The listing builds one solid part. Answer for the finished solid, in the listing's coordinates (mm). Face numbers are marked on the shaded views. A direction names the side the tool comes from. Give positions to 0.01 mm unless a question says otherwise; leave off trailing zeros. Order: outer loops, then holes, each group sorted by start corner. A loop starts at its lowest first (then second) coordinate and runs counter-clockwise, first axis right, second up. Notation, with made-up numbers: (64.25, 54) - (103.25, 54) arc R24 ccw to (103.25, 83) - close; hole circle Ø1 at (-9, 78.25). An arc over 180 degrees is marked (long way). Use CSV: the item, a comma, the result in double quotes.
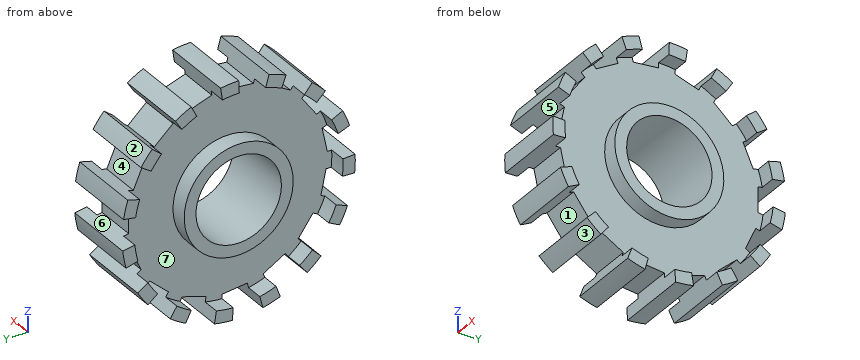
```python
from build123d import *

# Parameters (mm, degrees)
CUT_EXTRUDE3_DEPTH = 16
CIRPATTERN1_COUNT  = 15


with BuildPart() as part:
    # Sketch1 → Revolve1 (revolve)
    with BuildSketch(Plane.XY, mode=Mode.PRIVATE) as revolve1_sk:
        Polygon((0, 5.778414329), (-10, 5.778414329), (-10, 7.373034886), (-7.662379617, 7.373034886), (-7.662379617, 14.122184027), (-10, 14.122184027), (-10, 15.778414329), (0, 15.778414329), (0, 14.122184027), (-2.126486554, 14.122184027), (-2.126486554, 7.373034886), (0, 7.373034886), align=None)
    revolve(revolve1_sk.sketch.rotate(Axis((0, 0, 0), (-1, 0, 0)), 90), axis=Axis((0, 0, 0), (-1, 0, 0)))

    # Sketch2 → Cut-Extrude3 (cut)
    with BuildSketch(Plane(origin=(0, 0, 0), x_dir=(0, 0, -1), z_dir=(1, 0, 0))):
        Polygon((-2.776343501, 17.284448499), (-2.119655167, 13.369575739), (1.290072721, 13.369575739), (1.896246568, 17.284448499), align=None)
    cut_extrude3 = extrude(amount=-CUT_EXTRUDE3_DEPTH, mode=Mode.SUBTRACT)

    # CirPattern1: Cut-Extrude3 ×15 about axis
    cirpattern1_axis = Axis((0, 0, 0), (1, 0, 0))
    for i in range(1, CIRPATTERN1_COUNT):
        add(cut_extrude3.rotate(cirpattern1_axis, i * 360 / CIRPATTERN1_COUNT), mode=Mode.SUBTRACT)


solid = part.part
```
Item 1: The mould has two halves that part along Z. Classify the marked faces 1, 2 and 3: +Z half, -Z half, draft (parallel to the pull), parting line (faces both ways), or undercut.
Taken from the geometry:
face 1,"undercut"
face 2,"+Z half"
face 3,"-Z half"
Item 2: The part is cut by section A-A (z = 0). Give the vertices of the cut face in (x, y).
Taken from the geometry:
outline,"(-10, -15.78) - (0, -15.78) - (0, -14.12) - (-2.13, -14.12) - (-2.13, -7.37) - (0, -7.37) - (0, -5.78) - (-10, -5.78) - (-10, -7.37) - (-7.66, -7.37) - (-7.66, -14.12) - (-10, -14.12) - close; (-10, 5.78) - (0, 5.78) - (0, 7.37) - (-2.13, 7.37) - (-2.13, 13.37) - (-7.66, 13.37) - (-7.66, 7.37) - (-10, 7.37) - close"
Item 3: Each of these flat-tipped pins is pushed along its axis until it touches: pin 1 (10.5 mm diameter, centred on y = 0, z = 0, fed in from +X); pin 2 (3 mm diameter, centred on x = -4.5, z = -9, fed in from +Y); pin 3 (4 mm diameter, centred on y = -3, z = 4.5, fed in from -X); pin 4 (1 mm diameter, centred on x = -4, z = 1, fed in from +Y). Where does it stop, or does it pass through?
Taken from the geometry:
pin 1,"through"
pin 2,"y = 13.66"
pin 3,"x = -10"
pin 4,"y = 13.37"
Item 4: The part is cut by section C-C (z = 3.5). Give the vertices of the cut face in (x, y).
Taken from the geometry:
outline,"(-10, -6.49) - (-7.66, -6.49) - (-7.66, -12.92) - (-2.13, -12.92) - (-2.13, -6.49) - (0, -6.49) - (0, -4.6) - (-10, -4.6) - close; (-10, 4.6) - (0, 4.6) - (0, 6.49) - (-2.13, 6.49) - (-2.13, 13.68) - (0, 13.68) - (0, 15.39) - (-10, 15.39) - (-10, 13.68) - (-7.66, 13.68) - (-7.66, 6.49) - (-10, 6.49) - close"
Item 5: The part is cut by section B-B (x = -9). Count the separate pieces of the cut face and the enclosed holes in it, and give its area (3 significant figures).
Taken from the geometry:
separate pieces,"16"
enclosed holes,"1"
area,"125 mm^2"
Item 6: Find the intervals of material crossed by line 1 along Y through (x, z) = (-2, 0); line 2 along Y through (x, z) = (-7.5, 0); line 3 along Y through (x, z) = (-6.5, 14), in increasing order.
Taken from the geometry:
line 1,"-15.78 to -14.12, -7.37 to -5.78, 5.78 to 7.37"
line 2,"-15.78 to -5.78, 5.78 to 13.37"
line 3,"-6.26 to -3.76, -0.09 to 2.21, 6.21 to 7.28"
Item 7: Which of the six approach directions +Z, -Z, +X, -X, +Y, -Y give full straight-line access (tool end or side, diameter ignored) to the marked faces 4, 5, 6 and 7?
Taken from the geometry:
face 4,"+X, -X"
face 5,"+X, -X, -Y"
face 6,"+X, -X, +Y"
face 7,"-X"
